Build history of the part. All positions in model axes, mm. A direction names the side the tool comes from. Coordinates: 2 decimals unless noted, no trailing zeros. Order: outer loops, then holes, each group sorted by start corner. A loop starts at its lowest first (then second) coordinate and runs counter-clockwise, first axis right, second up. Notation, with made-up numbers: (-25, 78) - (-20, 78) arc R16 cw to (-20, 96) - close; hole circle Ø7 at (18.5, 59.5). An arc over 180 degrees is marked (long way). Return JSON: item names as keys, results as strings.
Autodesk Fusion 360 part; units mm, degrees
sketch "草图1" plane through (0, 0, 0) normal (0, 0, 1) x (1, 0, 0)
  circle A0 centre (0, 0) radius 14
  dimension "d1" = 28
extrude "拉伸1" add sketch "草图1" along normal blind 4 makes body 1
sketch "草图2" plane through (0, 0, 4) normal (0, 0, 1) x (-1, 0, 0)
  circle A0 centre (0, 0) radius 14
  circle A1 centre (0, 0) radius 11.5 construction
  line L0 (13, 0) -> (-13, 0)
  circle A2 centre (11.5, 0) radius 1.6
  circle A3 centre (-5.75, 9.9593) radius 1.6
  circle A4 centre (-5.75, -9.9593) radius 1.6
  circle A5 centre (0, 0) radius 10.5 construction
  circle A6 centre (-10.5, 0) radius 1.6
  circle A7 centre (5.25, -9.0933) radius 1.6
  circle A8 centre (5.25, 9.0933) radius 1.6
  dimension "d4" = 23
  dimension "d5" = 3.2
  dimension "d7" = 360
  dimension "d8" = 21
  dimension "d9" = 3.2
  dimension "d11" = 360
extrude "拉伸2" cut sketch "草图2" against normal blind 4 contours L0 A6 | L0 A6 | A2 | A3 | A4 | A7 | A8 bodies 1
sketch "草图3" plane through (0, 0, 4) normal (0, 0, 1) x (-1, 0, 0)
  circle A0 centre (-5.75, -9.9593) radius 1.6
  circle A1 centre (11.5, 0) radius 1.6
  circle A2 centre (-10.5, 0) radius 1.6
  circle A3 centre (5.25, 9.0933) radius 1.6
  circle A4 centre (5.25, -9.0933) radius 1.6
  circle A5 centre (-5.75, 9.9593) radius 1.6
  circle A6 centre (0, 0) radius 14
  circle A7 centre (0, 0) radius 7.5
  dimension "d14" = 15
extrude "拉伸3" add sketch "草图3" along normal blind 12 contours A7 bodies 1
sketch "草图4" plane through (0, 0, 16) normal (0, 0, 1) x (-1, 0, 0)
  circle A0 centre (0, 0) radius 7.5
  circle A1 centre (0, 0) radius 3
  dimension "d17" = 6
extrude "拉伸4" cut sketch "草图4" against normal blind 16 contours A1 bodies 1
ref_plane "工作平面1" through (0, 8, 0) normal (0, 1, 0) x (0, 0, 1)
sketch "草图5" plane through (0, 8, 0) normal (0, 1, 0) x (1, 0, 0)
  line L0 (0, -14) -> (0, 7)
  circle A0 centre (0, -8) radius 2
  dimension "d21" = 4
  dimension "d22" = 8
extrude "拉伸5" cut sketch "草图5" against normal blind 8 bodies 1
copy_body "实体->零部件1" bodies 1 removing the originals makes body 2 in component "Component'"
component "Component'" placed x (1, 0, 0) y (0, 1, 0) z (0, 0, 1) at (0, 0, 0)
1. Mould opens along X. For faces 3 (the cylindrical face through (1.63, -7.32, 9.92)), 4 (the cylindrical face through (-4.903, -7.531, 2.028)), 5 (the flat face through (6, -6, 4)) say: pulls with the +X half, pulls with the -X half, needs draft (parallel to the pull), parting line crosses it, or undercut.
Check values:
{"face 3": "parting line crosses it", "face 4": "undercut", "face 5": "needs draft"}
2. Cut at A-A on y = 0. Give the cut face in (x, z), plus the area to 3 significant figures.
Check values:
{"outline": "(-14, 0) - (-13.1, 0) - (-13.1, 4) - (-14, 4) - close; (-9.9, 0) - (-3, 0) - (-3, 16) - (-7.5, 16) - (-7.5, 4) - (-9.9, 4) - close; (3, 0) - (8.9, 0) - (8.9, 4) - (7.5, 4) - (7.5, 16) - (3, 16) - close; (12.1, 0) - (14, 0) - (14, 4) - (12.1, 4) - close", "area": "170 mm²"}
3. Tool access for faces 1 (the cylindrical face through (1.847, 4.905, 8.766)), 2 (the flat face through (-0.2, 3.3, 0)): list every direction of +Z, -Z, +X, -X, +Y, -Y with a clear straight run to the whole face (end or side of a thin tool).
Check values:
{"face 1": "+Y", "face 2": "-Z, +X, -X, +Y, -Y"}
4. Probe L1, parallel to Z at x = 0, y = 5.1; L2, parallel to Y at x = -5.25, z = 1.8; L3, parallel to Y at x = 10.5, z = 2.25. List the from-to ranges inside material, lowest first.
Check values:
{"L1": "0 to 6, 10 to 16", "L2": "-12.98 to -10.69, -7.49 to 7.49, 10.69 to 12.98", "L3": "-9.26 to -1.6, 1.6 to 9.26"}
5. Cut at D-D on z = 13.5. Give the cut face in (x, y).
Check values:
{"outline": "circle Ø15 at (0, 0); hole circle Ø6 at (0, 0)"}
6. Cut at C-C on x = -11.5. Give the cut face in (y, z).
Check values:
{"outline": "(-7.98, 0) - (-1.6, 0) - (-1.6, 4) - (-7.98, 4) - close; (1.6, 0) - (7.98, 0) - (7.98, 4) - (1.6, 4) - close"}
7. Drop flat-ended pins along their axis: pin 1 (3.5 mm diameter, centred on x = -11.5, y = 0, fed in from +Z); pin 2 (5.5 mm diameter, centred on x = 0, y = 0, fed in from -Z); pin 3 (3.5 mm diameter, centred on x = 0, z = 8, fed in from +Y); pin 4 (8 mm diameter, centred on x = -4, z = 8.5, fed in from +Y). Give the stop position or say it passes through.
Check values:
{"pin 1": "z = 4", "pin 2": "through", "pin 3": "y = -2.44", "pin 4": "y = 7.49"}
8. Cut at B-B on x = 0. Give the cut face in (y, z), plus the area to 3 significant figures.
Check values:
{"outline": "(-14, 0) - (-3, 0) - (-3, 16) - (-7.5, 16) - (-7.5, 4) - (-14, 4) - close; (3, 0) - (14, 0) - (14, 4) - (7.5, 4) - (7.5, 6) - (3, 6) - close; (3, 10) - (7.5, 10) - (7.5, 16) - (3, 16) - close", "area": "178 mm²"}
